```python
from build123d import *

# Parameters (mm, degrees)
SKETCH1_R           = 75
BOSS_EXTRUDE1_DEPTH = 5
SKETCH2_W           = 15
SKETCH2_H           = 4.5
CUT_EXTRUDE1_DEPTH  = 10
SKETCH3_R           = 2
CUT_EXTRUDE2_DEPTH  = 10


with BuildPart() as part:
    # Sketch1 → Boss-Extrude1 (new body)
    with BuildSketch(Plane(origin=(0, 0, 0), x_dir=(1, 0, 0), z_dir=(0, 1, 0))):
        with Locations(Location((0, 0, 0), (0, 0, 270))):
            Circle(SKETCH1_R)
    extrude(amount=BOSS_EXTRUDE1_DEPTH)

    # Sketch2 → Cut-Extrude1 (cut)
    with BuildSketch(Plane(origin=(0, 5, 0), x_dir=(1, 0, 0), z_dir=(0, 1, 0))):
        with Locations((-17.5, 47.25)):
            Rectangle(SKETCH2_W, SKETCH2_H)
        with Locations((17.5, 47.25)):
            Rectangle(SKETCH2_W, SKETCH2_H)
    cut_extrude1 = extrude(amount=-CUT_EXTRUDE1_DEPTH, mode=Mode.SUBTRACT)

    # Mirror1: Cut-Extrude1 across plane
    add(cut_extrude1.mirror(Plane.XY), mode=Mode.SUBTRACT)

    # Sketch3 → Cut-Extrude2 (cut)
    with BuildSketch(Plane(origin=(0, 5, 0), x_dir=(1, 0, 0), z_dir=(0, 1, 0))):
        with Locations(Location((0, 0, 0), (0, 0, 270))):
            Circle(SKETCH3_R)
    extrude(amount=-CUT_EXTRUDE2_DEPTH, mode=Mode.SUBTRACT)


solid = part.part
```
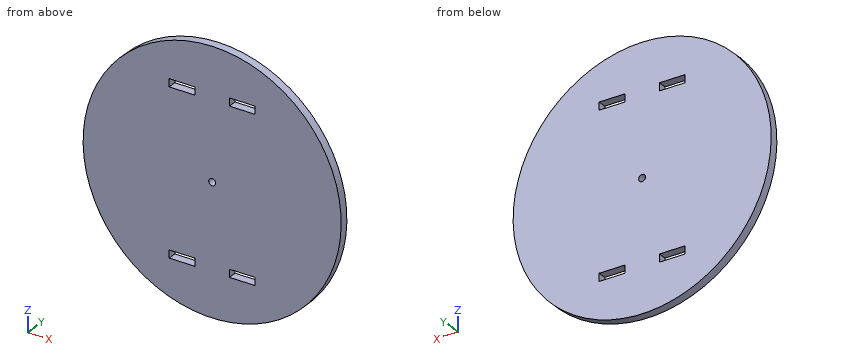
Model file for the job. Use its own axes, mm. Coordinates: 2 decimals unless noted, no trailing zeros. Order: outer loops, then holes, each group sorted by start corner. A loop starts at its lowest first (then second) coordinate and runs counter-clockwise, first axis right, second up. Notation, with made-up numbers: (-19.75, 13) -> (-8.75, 13) arc R18 ccw to (-8.75, 42) -> close; hole circle Ø6 at (86.5, 0). An arc over 180 degrees is marked (long way). Answer as a JSON object with one key per item and string values. Group by question number.
1) Flat gauge pins, fed straight in: pin 1 (1.3 mm diameter, centred on y = 1.5, z = 47.5, fed in from -X); pin 2 (2.5 mm diameter, centred on x = 17.5, y = 1.5, fed in from +Z); pin 3 (2.5 mm diameter, centred on x = 16.5, y = 1.5, fed in from -Z). Where does each tip first touch, or does it go through?
2) Drill centre lines: L1, parallel to X at y = 3.35, z = 0; L2, parallel to X at y = 3.1, z = -49; L3, parallel to Z at x = -20, y = 4.8. Where is each one in solid material? Low to high.
3) Cut at C-C, the plane y = 3. Write the cut outline in (x, z), then the cut area to 3 significant figures.
4) Cut at B-B, the plane x = 0. Write the cut outline in (y, z).
5) Cut at A-A, the plane z = 0. Write the cut outline in (x, y).
6) Cut at D-D, the plane z = 47.5. Write the cut outline in (x, y), then the cut area to 3 significant figures.
Check values:
{
 "1": {"pin 1": "stops at x = -58.57", "pin 2": "stops at z = 73.22", "pin 3": "stops at z = -73.43"},
 "2": {"L1": "x = -75 to -2, 2 to 75", "L2": "x = -56.78 to -25, -10 to 10, 25 to 56.78", "L3": "z = -72.28 to -49.5, -45 to 45, 49.5 to 72.28"},
 "3": {"outline": "circle Ø150 at (0, 0); hole (-25, -49.5) -> (-10, -49.5) -> (-10, -45) -> (-25, -45) -> close; hole (-25, 45) -> (-10, 45) -> (-10, 49.5) -> (-25, 49.5) -> close; hole circle Ø4 at (0, 0); hole (10, -49.5) -> (25, -49.5) -> (25, -45) -> (10, -45) -> close; hole (10, 45) -> (25, 45) -> (25, 49.5) -> (10, 49.5) -> close", "area": "17,400 mm²"},
 "4": {"outline": "(0, -75) -> (5, -75) -> (5, -2) -> (0, -2) -> close; (0, 2) -> (5, 2) -> (5, 75) -> (0, 75) -> close"},
 "5": {"outline": "(-75, 0) -> (-2, 0) -> (-2, 5) -> (-75, 5) -> close; (2, 0) -> (75, 0) -> (75, 5) -> (2, 5) -> close"},
 "6": {"outline": "(-58.04, 0) -> (-25, 0) -> (-25, 5) -> (-58.04, 5) -> close; (-10, 0) -> (10, 0) -> (10, 5) -> (-10, 5) -> close; (25, 0) -> (58.04, 0) -> (58.04, 5) -> (25, 5) -> close", "area": "430 mm²"}
}
